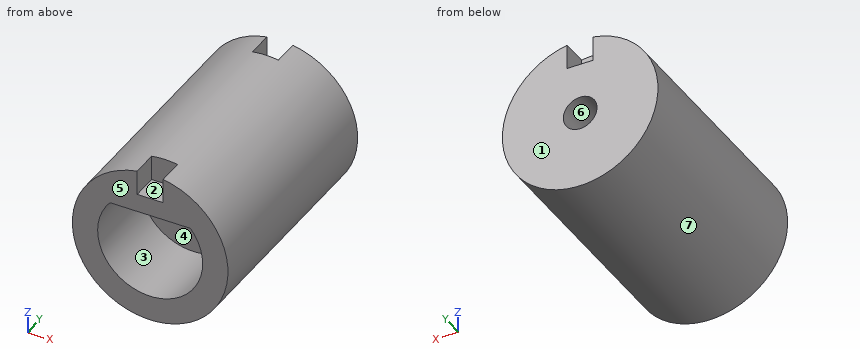
from build123d import *

# Parameters (mm, degrees)
ESBO_O2_R                = 6
ESBO_O2_R_2              = 1.3
RESSALTO_EXTRUS_O1_DEPTH = 9
CORTE_EXTRUS_O1_DEPTH    = 6
ESBO_O4_W                = 2
ESBO_O4_H                = 3
CORTE_EXTRUS_O2_DEPTH    = 2


with BuildPart() as part:
    # Esboço2 → Ressalto-extrusão1 (new, symmetric)
    with BuildSketch(Plane(origin=(0, 0, 0), x_dir=(1, 0, 0), z_dir=(0, 1, 0))):
        with Locations(Location((0, 0, 0), (0, 0, 270))):
            Circle(ESBO_O2_R)
        with Locations(Location((0, 0, 0), (0, 0, 270))):
            Circle(ESBO_O2_R_2, mode=Mode.SUBTRACT)
    extrude(amount=RESSALTO_EXTRUS_O1_DEPTH, both=True)

    # Esboço3 → Corte-extrusão1 (cut)
    with BuildSketch(Plane.XZ.offset(9)):
        with BuildLine():
            Line((-3.105237511, 2.6), (3.105237511, 2.6))
            ThreePointArc((3.105237511, 2.6), (0, -4.05), (-3.105237511, 2.6))
        make_face()
    extrude(amount=-CORTE_EXTRUS_O1_DEPTH, mode=Mode.SUBTRACT)

    # Esboço4 → Corte-extrusão2 (cut)
    with BuildSketch(Plane(origin=(0, 9, 0), x_dir=(1, 0, 0), z_dir=(0, 1, 0))):
        with Locations((0, -5.5)):
            Rectangle(ESBO_O4_W, ESBO_O4_H)
    corte_extrus_o2 = extrude(amount=-CORTE_EXTRUS_O2_DEPTH, mode=Mode.SUBTRACT)

    # Espelhar1: Corte-extrusão2 across plane
    add(corte_extrus_o2.mirror(Plane.ZX), mode=Mode.SUBTRACT)


solid = part.part
Build history of the part. All positions in model axes, mm. Face numbers are marked on the shaded views. A direction names the side the tool comes from. Round coordinates to 2 decimals unless told otherwise and drop trailing zeros. Write each loop counter-clockwise with the first axis right and the second up, starting at its lowest first coordinate (ties: lowest second). Pieces come first, ordered by that corner, then holes. Notation, with made-up numbers: M -35.5,78 L 22.5,78 A30 ccw 22.5,101 Z; hole C -25,67 d1. An arc over 180 degrees is marked long. Answer in a Markdown table with one row per item.
1. Flat gauge pins, fed straight in: P1, Ø4, axis at y = 2.5, z = 2.5, coming from the +X side; P2, Ø2, axis at y = 7.5, z = 5, coming from the -X side; P3, Ø3.5, axis at x = 0, z = 0, coming from the -Y side. Where does each tip first touch, or does it go through?
Geometry check:
| item | result |
|---|---|
| P1 | x = 5.98 |
| P2 | x = -4.47 |
| P3 | y = -3 |
2. Which spindle directions (+Z, -Z, +X, -X, +Y, -Y) get a long thin tool onto all of the face, cutting with end or side? Do the marked faces 1, 2 and 3. Say none if no direction does.
Geometry check:
| item | result |
|---|---|
| face 1 | +Z, -Z, +X, -X, +Y |
| face 2 | +Z, -Y |
| face 3 | -Y |
3. Saw through at A-A (z = 0). List the corners of the cut face in (x, y), and give its area (3 significant figures).
Geometry check:
| item | result |
|---|---|
| outline | M -6,-9 L -4.05,-9 L -4.05,-3 L -1.3,-3 L -1.3,9 L -6,9 Z; M 1.3,-3 L 4.05,-3 L 4.05,-9 L 6,-9 L 6,9 L 1.3,9 Z |
| area | 136 mm2 |
4. Mould opens along X. For the marked faces 4, 5, 6 and 7 say: +X half, -X half, draft (parallel to the pull), parting line (faces both ways), or undercut.
Geometry check:
| item | result |
|---|---|
| face 4 | undercut |
| face 5 | draft |
| face 6 | undercut |
| face 7 | parting line |
5. Probe L1, parallel to Z at x = 0, y = -6; L2, parallel to Z at x = 0, y = 5; L3, parallel to Y at x = 1.75, z = -3. List the from-to ranges inside material, lowest first. Write a range as [from, to].
Geometry check:
| item | result |
|---|---|
| L1 | [-6, -4.05], [2.6, 6] |
| L2 | [-6, -1.3], [1.3, 6] |
| L3 | [-3, 9] |
6. Saw through at C-C (y = 7.75). List the corners of the cut face in (x, z).
Geometry check:
| item | result |
|---|---|
| outline | M -1,4 L -1,5.92 A6 ccw long 1,5.92 L 1,4 Z; hole C 0,0 d2.6 |
7. Saw through at B-B (x = 0). List the corners of the cut face in (y, z).
Geometry check:
| item | result |
|---|---|
| outline | M -9,-6 L 9,-6 L 9,-1.3 L -3,-1.3 L -3,-4.05 L -9,-4.05 Z; M -9,2.6 L -3,2.6 L -3,1.3 L 9,1.3 L 9,4 L 7,4 L 7,6 L -7,6 L -7,4 L -9,4 Z |
8. Saw through at D-D (z = -3.75). List the corners of the cut face in (x, y), and give its area (3 significant figures).
Geometry check:
| item | result |
|---|---|
| outline | M -4.68,-9 L -1.53,-9 L -1.53,-3 L 1.53,-3 L 1.53,-9 L 4.68,-9 L 4.68,9 L -4.68,9 Z |
| area | 150 mm2 |
